Can you work these out from the drawing? Everything is in mm from the part's minimum corner. Coordinates: 2 decimals unless noted, no trailing zeros. Order: outer loops, then holes, each group sorted by start corner. A loop starts at its lowest first (then second) coordinate and runs counter-clockwise, first axis right, second up. Notation, with made-up numbers: (-29.75, -27) -> (14.25, -27) arc R22 cw to (14.25, 11) -> close; hole circle Ø5 at (61.25, -36.75). An arc over 180 degrees is marked (long way). Write item = value, one per line. Start each with the question number.
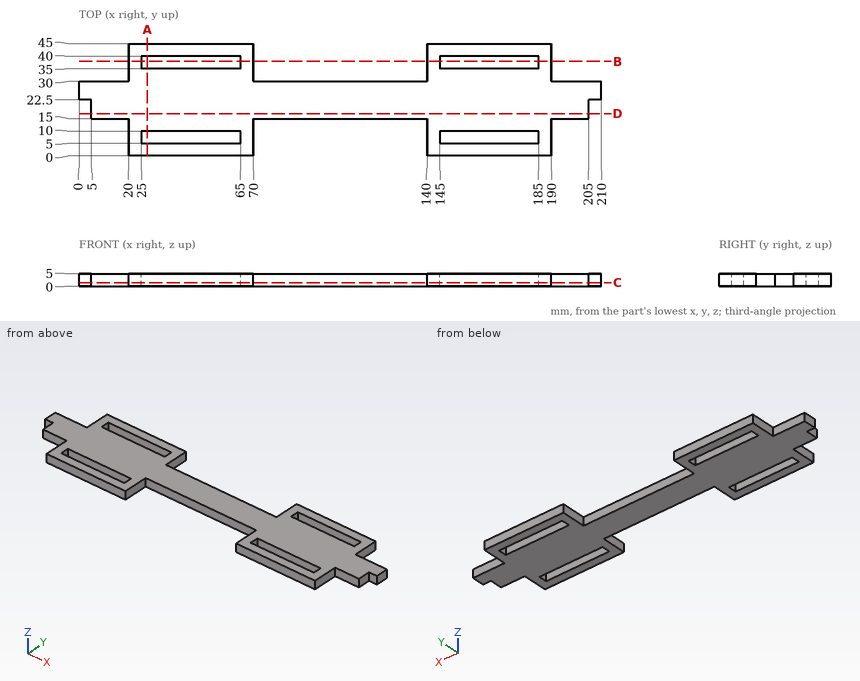
(1) Imagine slicing it at A-A (x = 27.5). Write out the boundary of the cut face in (y, z).
(2) Imagine slicing it at C-C (z = 1.5). Count the separate pieces of the cut face and the enclosed holes in it, plus the area to 4 significant figures.
(3) If I drill on L1, parallel to X at y = 6, z = 1.85; L2, parallel to Y at x = 161.5, z = 0.4; L3, parallel to X at y = 43, z = 2.4, over which ranges is the centre line in solid material (lowest first)? Write a range as from..to.
(4) Imagine slicing it at D-D (y = 17). Write out the boundary of the cut face in (x, z), plus the area to 3 significant figures.
(5) For P1, Ø2.5, axis at y = 38.5, z = 3, coming from the -X side; P2, Ø2.5, axis at y = 20, z = 2, coming from the +X side; P3, Ø2.5, axis at x = 208.5, z = 1.5, coming from the -Y side; P4, Ø1.5, axis at x = 169, z = 2.5, coming from the -Y side, each with a flat end and sliding along its axis, tell me the tip position at first contact or that it passes through.
(6) Imagine slicing it at B-B (y = 38). Write out the boundary of the cut face in (x, z), plus the area to 3 significant figures.
Result set:
q1.outline = (0, 0) -> (5, 0) -> (5, 5) -> (0, 5) -> close; (10, 0) -> (35, 0) -> (35, 5) -> (10, 5) -> close; (40, 0) -> (45, 0) -> (45, 5) -> (40, 5) -> close
q2.separate_pieces = 1
q2.enclosed_holes = 4
q2.area = 5,275 mm2
q3.L1 = 20..25, 65..70, 140..145, 185..190
q3.L2 = 0..5, 10..35, 40..45
q3.L3 = 20..70, 140..190
q4.outline = (5, 0) -> (205, 0) -> (205, 5) -> (5, 5) -> close
q4.area = 1,000 mm2
q5.P1 = 20
q5.P2 = 205
q5.P3 = 22.5
q5.P4 = 0
q6.outline = (20, 0) -> (25, 0) -> (25, 5) -> (20, 5) -> close; (65, 0) -> (70, 0) -> (70, 5) -> (65, 5) -> close; (140, 0) -> (145, 0) -> (145, 5) -> (140, 5) -> close; (185, 0) -> (190, 0) -> (190, 5) -> (185, 5) -> close
q6.area = 100 mm2
